For this review, take the finished solid that the model builds, in its own axes (mm). A direction names the side the tool comes from. Round coordinates to 2 decimals unless told otherwise and drop trailing zeros. Loops run counter-clockwise (first coordinate to the right, second up) from the corner with the lowest first, then second, coordinate; pieces in that order, holes last.
1) Take a section at D-D (y = 22.5). State the section outline as (x, z) points (1 decimal), then the cut area to 3 significant figures.
2) Mouldability with a two-part tool opening along X and no side actions: class faces 5 (the cylindrical face through (4.336, -1.479, -19.524)), 6 (the cylindrical face through (23.319, 14.196, 19.753)), 7 (the flat face through (47, 27, 0)) as pulls with the +X half, pulls with the -X half, needs draft (parallel to the pull), parting line crosses it, or undercut.
3) Take a section at A-A (x = 0). State the section outline as (y, z) points.
4) Insertion check: pin 1 (12 mm diameter, centred on y = 7.5, z = 29, fed in from -X); pin 2 (7 mm diameter, centred on x = 22.27, z = 22.27, fed in from -Y); pin 3 (2 mm diameter, centred on y = 5.5, z = 14.5, fed in from -X); pin 4 (3 mm diameter, centred on x = 0, z = -29.5, fed in from +Y). Each pin has a flat end and moves straight along its axis. Give the tip position at first contact, or say it passes through.
5) Take a section at C-C (z = 0). State the section outline as (x, y) points.
6) Tool access review of faces 1 (the flat face through (44, 13, 25)), 2 (the flat face through (20, 0, 9)), 3 (the cylindrical face through (-21.23, 14.2, 19.75)), 4 (the flat face through (44, 13, -25)): name each direction out of +Z, -Z, +X, -X, +Y, -Y from which nothing blocks a thin tool from reaching the whole face with its end or side.
7) Wall thickness on L1, parallel to Z at x = 0, y = 10; L2, parallel to Z at x = 22.5, y = 13.5; L3, parallel to X at y = 22, z = 1: over which ranges is each line inside the solid? List them lowest first.
8) Take a section at B-B (z = -31). State the section outline as (x, y) points.
Autodesk Inventor part; units mm, degrees
ref_plane "YZ Plane" through (0, 0, 0) normal (1, 0, 0) x (0, 1, 0)
ref_plane "XZ Plane" through (0, 0, 0) normal (0, 1, 0) x (-1, 0, 0)
ref_plane "XY Plane" through (0, 0, 0) normal (0, 0, 1) x (1, 0, 0)
sketch "Sketch1" plane through (0, 0, 0) normal (0, 1, 0) x (-1, 0, 0)
  circle A0 centre (0, 0) radius 40
  circle A1 centre (0, 0) radius 20
  line L0 (-57, 25) -> (-31.225, 25)
  line L1 (-31.225, -25) -> (-57, -25)
  line L2 (-57, -25) -> (-57, 25)
  point P0 (22.2739, 22.2739)
  point P1 (-22.2739, 22.2739)
  point P2 (-22.2739, -22.2739)
  point P3 (22.2739, -22.2739)
  dimension "d0" = 80
  dimension "d2" = 40
  dimension "d5" = 97
  dimension "d6" = 50
  dimension "d7" = 31.5
  dimension "d10" = 360
extrude "Extrusion1" add sketch "Sketch1" along normal blind 28 contours A0
extrude "Extrusion2" add sketch "Sketch1" along normal blind 28 contours A1
extrude "Extrusion3" add sketch "Sketch1" against normal blind 3 contours A1
extrude "Extrusion4" add sketch "Sketch1" along normal blind 27 contours A0 L1 L2 L0
hole "Hole1" at (-22.2739, 0, 22.2739) at (22.2739, 0, 22.2739) at (22.2739, 0, -22.2739) at (-22.2739, 0, -22.2739) direction (0, 1, 0) diameter 5.459 end through all
sketch "Sketch2" plane through (0, 28, 0) normal (0, 1, 0) x (1, 0, 0)
  circle A0 centre (0, 0) radius 40
  point P0 (0, 31.5)
  point P1 (0, -31.5)
  dimension "d27" = 31.5
  dimension "d30" = 360
hole "Hole2" at (0, 28, 31.5) at (0, 28, -31.5) direction (0, -1, 0) diameter 6.6 end through all
properties part number "CFS080CA501U"
Response:
1. outline: (31.2, -25) - (57, -25) - (57, 25) - (31.2, 25) arc R40 ccw (long way) to start; hole circle Ø5.5 at (-22.3, -22.3); hole circle Ø5.5 at (-22.3, 22.3); hole circle Ø6.6 at (0, -31.5); hole circle Ø6.6 at (0, 31.5); hole circle Ø5.5 at (22.3, -22.3); hole circle Ø5.5 at (22.3, 22.3)
1. area: 5,850 mm2
2. face 5: parting line crosses it
2. face 6: undercut
2. face 7: needs draft
3. outline: (-3, -20) - (0, -20) - (0, -28.2) - (28, -28.2) - (28, 28.2) - (0, 28.2) - (0, 20) - (-3, 20) - close; (0, -40) - (28, -40) - (28, -34.8) - (0, -34.8) - close; (0, 34.8) - (28, 34.8) - (28, 40) - (0, 40) - close
4. pin 1: stops at x = -32.73
4. pin 2: stops at y = 0
4. pin 3: stops at x = -37.65
4. pin 4: stops at y = 28
5. outline: (-40, 0) - (-20, 0) - (-20, -3) - (20, -3) - (20, 0) - (57, 0) - (57, 27) - (40, 27) - (40, 28) - (-40, 28) - close
6. face 1: +Z, +X, +Y, -Y
6. face 2: -Y
6. face 3: +Y, -Y
6. face 4: -Z, +X, +Y, -Y
7. L1: z = -40 to -34.8, -28.2 to 28.2, 34.8 to 40
7. L2: z = -33.07 to -24.99, -19.55 to 19.55, 24.99 to 33.07
7. L3: x = -39.99 to 57
8. outline: (-25.28, 0) - (-3.26, 0) - (-3.26, 28) - (-25.28, 28) - close; (3.26, 0) - (25.28, 0) - (25.28, 28) - (3.26, 28) - close
